Design review of the part built by this model. Coordinates are the model's own, in mm. Coordinates: 2 decimals unless noted, no trailing zeros. Write each loop counter-clockwise with the first axis right and the second up, starting at its lowest first coordinate (ties: lowest second). Pieces come first, ordered by that corner, then holes.
Q1. The part is to be moulded in two halves that separate along X. For faces 1 (the cylindrical face through (100.19, 1.61, -192.38)), 2 (the flat face through (113, 3.175, -142)), say which applies: released by +X, released by -X, zero draft, split by the parting line, or undercut.
Q2. For pin 1 Ø2 at (x, z) = (61.34, -73.42) entering from -Y, flat-tipped, find the tip position at first contact; note if it passes through.
Q3. Take a section at B-B, the plane x = 202.5. Write out the cut boundary in (y, z) (3 decimals).
Q4. For L1, parallel to X at y = 2.8, z = -22; L2, parallel to Z at x = 94.75, y = 1.35; L3, parallel to Z at x = 215.5, y = 3.05, list the stretches that pass through material, from the lowest coordinate up.
Q5. Take a section at C-C, the plane y = 1.45. State how many separate pieces and enclosed holes the cut face has, plus the area to 3 significant figures.
Q6. Take a section at A-A, the plane z = -59.5. Write out the cut boundary in (x, y) (3 decimals), plus the area to 3 significant figures.
from build123d import *

# Parameters (mm, degrees)
SKETCH1_W               = 228.6
SKETCH1_H               = 279.4
BOSS_EXTRUDE1_DEPTH     = 3.175
SKETCH3_R               = 1.7
SKETCH3_W               = 25.4
SKETCH3_H               = 88.9
CUT_EXTRUDE1_DEPTH      = 4.175
SKETCH4_R               = 17.78
SKETCH4_R_2             = 2.25
CUT_EXTRUDE2_DEPTH      = 4.175
SKETCH5_R               = 1.75
CUT_EXTRUDE3_DEPTH      = 4.175
SKETCH6_R               = 1.25
CUT_EXTRUDE4_DEPTH      = 4.175
SKETCH7_R               = 1.75
CUT_EXTRUDE5_DEPTH      = 4.175
SKETCH8_R               = 1.726999975
SKETCH8_R_2             = 6.35
CUT_EXTRUDE6_DEPTH      = 1
CUT_EXTRUDE6_DEPTH_BACK = 4.175
SKETCH10_W              = 75.000000114
SKETCH10_H              = 14.999999972
BOSS_EXTRUDE2_DEPTH     = 3.175
SKETCH9_R               = 1.599999975
SKETCH9_W               = 29.999999944
SKETCH9_H               = 13.700000032
CUT_EXTRUDE7_DEPTH      = 1
CUT_EXTRUDE7_DEPTH_BACK = 4.175


with BuildPart() as part:
    # Sketch1 → Boss-Extrude1 (new body)
    with BuildSketch(Plane(origin=(0, 0, 0), x_dir=(1, 0, 0), z_dir=(0, 1, 0))):
        with Locations((114.3, 139.7)):
            Rectangle(SKETCH1_W, SKETCH1_H)
    extrude(amount=BOSS_EXTRUDE1_DEPTH)

    # Sketch3 → Cut-Extrude1 (cut, through all)
    with BuildSketch(Plane(origin=(0, 3.175, 0), x_dir=(1, 0, 0), z_dir=(0, 1, 0))):
        with Locations((85.34, 43.42)):
            Circle(SKETCH3_R)
        with Locations((61.34, 43.42)):
            Circle(SKETCH3_R)
        with Locations((85.34, 73.42)):
            Circle(SKETCH3_R)
        with Locations((61.34, 73.42)):
            Circle(SKETCH3_R)
        with Locations((167.26, 73.42)):
            Circle(SKETCH3_R)
        with Locations((143.26, 73.42)):
            Circle(SKETCH3_R)
        with Locations((167.26, 43.42)):
            Circle(SKETCH3_R)
        with Locations((143.26, 43.42)):
            Circle(SKETCH3_R)
        with Locations((203.2, 58.42)):
            Rectangle(SKETCH3_W, SKETCH3_H)
        with Locations((25.4, 58.42)):
            Rectangle(SKETCH3_W, SKETCH3_H)
    extrude(amount=-CUT_EXTRUDE1_DEPTH, mode=Mode.SUBTRACT)

    # Sketch4 → Cut-Extrude2 (cut, through all)
    with BuildSketch(Plane(origin=(0, 3.175, 0), x_dir=(1, 0, 0), z_dir=(0, 1, 0))):
        with Locations((114.3, 203.2)):
            Circle(SKETCH4_R)
        with Locations((114.3, 224.79)):
            Circle(SKETCH4_R_2)
        with Locations((114.3, 181.61)):
            Circle(SKETCH4_R_2)
    extrude(amount=-CUT_EXTRUDE2_DEPTH, mode=Mode.SUBTRACT)

    # Sketch5 → Cut-Extrude3 (cut, through all)
    with BuildSketch(Plane(origin=(0, 3.175, 0), x_dir=(1, 0, 0), z_dir=(0, 1, 0))):
        with Locations((90.5, 198.41)):
            Circle(SKETCH5_R)
        with Locations((90.5, 109.41)):
            Circle(SKETCH5_R)
        with Locations((4, 109.41)):
            Circle(SKETCH5_R)
        with Locations((4, 198.41)):
            Circle(SKETCH5_R)
    extrude(amount=-CUT_EXTRUDE3_DEPTH, mode=Mode.SUBTRACT)

    # Sketch6 → Cut-Extrude4 (cut, through all)
    with BuildSketch(Plane(origin=(0, 3.175, 0), x_dir=(1, 0, 0), z_dir=(0, 1, 0))):
        with Locations((154.25, 247.102093509)):
            Circle(SKETCH6_R)
        with Locations((220.25, 247.102093509)):
            Circle(SKETCH6_R)
        with Locations((220.25, 201.102093509)):
            Circle(SKETCH6_R)
        with Locations((154.25, 201.102093509)):
            Circle(SKETCH6_R)
        with Locations((220.25, 192.022093509)):
            Circle(SKETCH6_R)
        with Locations((220.25, 146.022093509)):
            Circle(SKETCH6_R)
        with Locations((154.25, 146.022093509)):
            Circle(SKETCH6_R)
        with Locations((154.25, 192.022093509)):
            Circle(SKETCH6_R)
    extrude(amount=-CUT_EXTRUDE4_DEPTH, mode=Mode.SUBTRACT)

    # Sketch7 → Cut-Extrude5 (cut, through all)
    with BuildSketch(Plane(origin=(0, 3.175, 0), x_dir=(1, 0, 0), z_dir=(0, 1, 0))):
        with Locations((127.38, 134.915)):
            Circle(SKETCH7_R)
        with Locations((170.62, 134.915)):
            Circle(SKETCH7_R)
        with Locations((119.38, 86.675)):
            Circle(SKETCH7_R)
        with Locations((182.82, 86.675)):
            Circle(SKETCH7_R)
    extrude(amount=-CUT_EXTRUDE5_DEPTH, mode=Mode.SUBTRACT)

    # Sketch8 → Cut-Extrude6 (cut, two sides)
    with BuildSketch(Plane(origin=(0, 3.175, 0), x_dir=(1, 0, 0), z_dir=(0, 1, 0))) as cut_extrude6_sk:
        with Locations((20.63749043, 258.7625)):
            Circle(SKETCH8_R)
        with Locations((4.76249043, 258.7625)):
            Circle(SKETCH8_R)
        with Locations((4.76249043, 274.6375)):
            Circle(SKETCH8_R)
        with Locations((20.63749043, 274.6375)):
            Circle(SKETCH8_R)
        with Locations((12.69999043, 266.7)):
            Circle(SKETCH8_R_2)
        with Locations((58.10249043, 14.2875)):
            Circle(SKETCH8_R)
        with Locations((73.97749043, 14.2875)):
            Circle(SKETCH8_R)
        with Locations((66.03999043, 22.225)):
            Circle(SKETCH8_R_2)
        with Locations((58.10249043, 30.1625)):
            Circle(SKETCH8_R)
        with Locations((73.97749043, 30.1625)):
            Circle(SKETCH8_R)
        with Locations((170.49749043, 14.2875)):
            Circle(SKETCH8_R)
        with Locations((154.62249043, 14.2875)):
            Circle(SKETCH8_R)
        with Locations((154.62249043, 30.1625)):
            Circle(SKETCH8_R)
        with Locations((170.49749043, 30.1625)):
            Circle(SKETCH8_R)
        with Locations((162.55999043, 22.225)):
            Circle(SKETCH8_R_2)
        with Locations((106.36249043, 150.8125)):
            Circle(SKETCH8_R)
        with Locations((122.23749043, 150.8125)):
            Circle(SKETCH8_R)
        with Locations((114.29999043, 158.75)):
            Circle(SKETCH8_R_2)
        with Locations((106.36249043, 166.6875)):
            Circle(SKETCH8_R)
        with Locations((122.23749043, 166.6875)):
            Circle(SKETCH8_R)
        with Locations((223.83749043, 258.7625)):
            Circle(SKETCH8_R)
        with Locations((207.96249043, 258.7625)):
            Circle(SKETCH8_R)
        with Locations((207.96249043, 274.6375)):
            Circle(SKETCH8_R)
        with Locations((223.83749043, 274.6375)):
            Circle(SKETCH8_R)
        with Locations((215.89999043, 266.7)):
            Circle(SKETCH8_R_2)
    extrude(amount=CUT_EXTRUDE6_DEPTH, mode=Mode.SUBTRACT)
    extrude(cut_extrude6_sk.sketch, amount=-CUT_EXTRUDE6_DEPTH_BACK, mode=Mode.SUBTRACT)

    # Sketch10 → Boss-Extrude2 (add)
    with BuildSketch(Plane.XZ):
        with Locations((114.3, 7.499999986)):
            Rectangle(SKETCH10_W, SKETCH10_H)
        with Locations((114.3, -286.899999986)):
            Rectangle(SKETCH10_W, SKETCH10_H)
    extrude(amount=-BOSS_EXTRUDE2_DEPTH)

    # Sketch9 → Cut-Extrude7 (cut, two sides)
    with BuildSketch(Plane(origin=(0, 3.175, 0), x_dir=(1, 0, 0), z_dir=(0, 1, 0))) as cut_extrude7_sk:
        with Locations((133.850000016, 287.549999984)):
            Circle(SKETCH9_R)
        with Locations((94.749999984, 287.549999984)):
            Circle(SKETCH9_R)
        with Locations((133.850000016, -8.149999984)):
            Circle(SKETCH9_R)
        with Locations((94.749999984, -8.149999984)):
            Circle(SKETCH9_R)
        with Locations((114.3, 287.549999984)):
            Rectangle(SKETCH9_W, SKETCH9_H)
        with Locations((114.3, -8.149999984)):
            Rectangle(SKETCH9_W, SKETCH9_H)
    extrude(amount=CUT_EXTRUDE7_DEPTH, mode=Mode.SUBTRACT)
    extrude(cut_extrude7_sk.sketch, amount=-CUT_EXTRUDE7_DEPTH_BACK, mode=Mode.SUBTRACT)


solid = part.part
Responses:
1. face 1: undercut
1. face 2: zero draft
2. pin 1: passes through
3. outline: (0, -279.4) - (3.175, -279.4) - (3.175, -102.87) - (0, -102.87) - close; (0, -13.97) - (3.175, -13.97) - (3.175, 0) - (0, 0) - close
4. L1: x = 0 to 12.7, 38.1 to 59.69, 72.39 to 156.21, 168.91 to 190.5, 215.9 to 228.6
4. L2: z = -294.4 to -289.15, -285.95 to 6.55, 9.75 to 15
4. L3: z = -279.4 to -273.04, -260.36 to -102.87, -13.97 to 0
5. separate pieces: 1
5. enclosed holes: 58
5. area: 58,700 mm2
6. outline: (0, 0) - (12.7, 0) - (12.7, 3.175) - (0, 3.175) - close; (38.1, 0) - (190.5, 0) - (190.5, 3.175) - (38.1, 3.175) - close; (215.9, 0) - (228.6, 0) - (228.6, 3.175) - (215.9, 3.175) - close
6. area: 565 mm2
